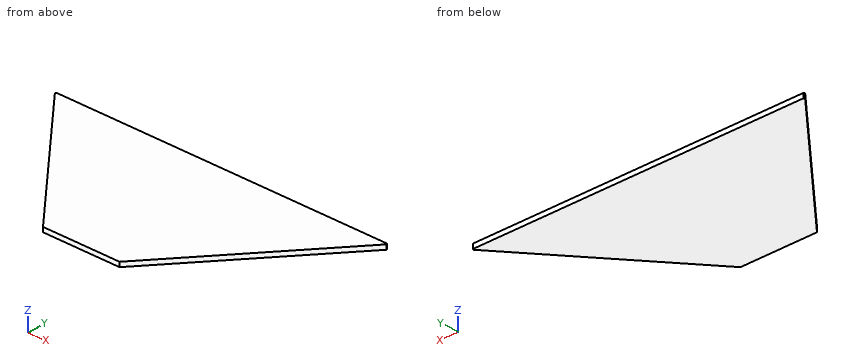
Autodesk Inventor part; units mm, degrees
ref_plane "YZ Plane" through (0, 0, 0) normal (1, 0, 0) x (0, 1, 0)
ref_plane "XZ Plane" through (0, 0, 0) normal (0, 1, 0) x (-1, 0, 0)
ref_plane "XY Plane" through (0, 0, 0) normal (0, 0, 1) x (1, 0, 0)
sketch "Sketch1" plane through (0, 0, 0) normal (0, 0, 1) x (1, 0, 0)
  line L0 (-108.91, 100) -> (-25, 0)
  line L1 (-25, 0) -> (25, 0)
  line L2 (25, 0) -> (108.91, 100)
  line L3 (108.91, 100) -> (-108.91, 100)
  point P0 (0, 0)
  point P1 (0, 0)
  point P2 (0, 100)
  dimension "BendRadius" = 3
  dimension "d0" = 100
  dimension "d1" = 50
  dimension "d2" = 217.8199
  dimension "d4" = 130
extrude "Plate1" add sketch "Sketch1" along normal blind 3
chamfer "Chamfer1" distance 1 angle 45 2 edges at (-108.91, 100, 1.5) (108.91, 100, 1.5)
equation "\"BendRadius\" = Thickness"
equation "\"d0\" = Лоток_высота"
equation "\"d1\" = Лоток_ширина_низ"
equation "\"d4\" = Лоток_угол"
equation "\"d3\" = Thickness"
equation "\"BendReliefWidth\" = Thickness"
equation "\"BendReliefDepth\" = 0.5 * Thickness"
equation "\"CornerReliefSize\" = 4 * Thickness"
equation "\"MinimumRemnant\" = 2 * Thickness"
equation "\"TransitionRadius\" = BendRadius"
equation "\"JacobiRadiusSize\" = BendRadius"
equation "\"GapSize\" = Thickness"
properties part number "ДМС 304 торец лотка кормовой"
Verification items for the finished model (mm, model axes). Coordinates: 2 decimals unless noted, no trailing zeros. Order: outer loops, then holes, each group sorted by start corner. A loop starts at its lowest first (then second) coordinate and runs counter-clockwise, first axis right, second up. Notation, with made-up numbers: (54.25, 63.5) -> (80.25, 63.5) arc R11 ccw to (80.25, 67.5) -> close; hole circle Ø11 at (49, 49). An arc over 180 degrees is marked (long way). Use CSV: the item, a comma, the result in double quotes. Start each with the question number.
Q1. Thickness scan on line 1 along Y through (x, z) = (72.5, 2); line 2 along Y through (x, z) = (36.5, 1.8); line 3 along X through (y, z) = (89, 2.55). Record the ranges inside material, lowest first.
Q2. Depth check by flat-ended pin: P1, Ø1.5, axis at y = 24.5, z = 1, coming from the -X side. Enter the tip coordinate at first touch or a pass-through.
Q3. Section check A-A, the plane z = 1.7. Record the cut outline in (x, y), and give its area (3 significant figures).
Q4. Section check B-B, the plane y = 90. Record the cut outline in (x, z).
Q5. Section check C-C, the plane x = -39.5. Record the cut outline in (y, z).
Returned:
1,line 1,"y = 56.61 to 100"
1,line 2,"y = 13.71 to 100"
1,line 3,"x = -99.68 to 99.68"
2,P1,"stops at x = -46.19"
3,outline,"(-108.27, 99.23) -> (-25, 0) -> (25, 0) -> (108.27, 99.23) -> (107.91, 100) -> (-107.91, 100) -> close"
3,area,"13,400 mm^2"
4,outline,"(-100.52, 0) -> (100.52, 0) -> (100.52, 3) -> (-100.52, 3) -> close"
5,outline,"(17.28, 0) -> (100, 0) -> (100, 3) -> (17.28, 3) -> close"
